Geometry: final body of the model. Coordinates: model frame, mm. A direction names the side the tool comes from. Give positions to 0.01 mm unless a question says otherwise; leave off trailing zeros. Loops run counter-clockwise (first coordinate to the right, second up) from the corner with the lowest first, then second, coordinate; pieces in that order, holes last. Notation, with made-up numbers: (-14, -25) -> (40, -25) arc R28 ccw to (40, 8) -> close; hole circle Ø6 at (-38, 28.5). An arc over 180 degrees is marked (long way). Answer in a Markdown table with one row per item. Add a question column.
1) Line query: line 1 (X direction, y = 10, z = 15.5); line 2 (X direction, y = 3.5, z = 10.25); line 3 (Y direction, x = -108.75, z = 9.75). Output: solid intervals per line, ascending. Write a range as from..to.
2) First-contact query: P1, Ø3, axis at x = -49, y = 33.5, coming from the -Z side; P2, Ø4.5, axis at x = -108.75, y = 10, coming from the +Z side; P3, Ø8, axis at x = -129.5, z = 9.5, coming from the +Y side. Flat tips, straight axial feed; report the tip coordinate or a pass-through.
3) Section query A-A (z = 1.75). Return the cut outline in (x, y), plus the area to 3 significant figures.
4) Section query B-B (x = -108.75). Return the cut outline in (y, z), plus the area to 3 significant figures.
5) Access query for faces 1 (the flat face through (-74, 0, 10)), 2 (the cylindrical face through (-92.73, 0.52, 10.14)). Directions: +Z, -Z, +X, -X, +Y, -Y. A direction counts if a zero-diameter tool reaches every point of the face in a straight line with its end or side. Return the directions, or none.
6) Section query C-C (y = 25). Return the cut outline in (x, z).
7) Section query D-D (x = -40). Return the cut outline in (y, z).
Autodesk Inventor part; units mm, degrees
ref_plane "YZ Plane" through (0, 0, 0) normal (1, 0, 0) x (0, 1, 0)
ref_plane "XZ Plane" through (0, 0, 0) normal (0, 1, 0) x (-1, 0, 0)
ref_plane "XY Plane" through (0, 0, 0) normal (0, 0, 1) x (1, 0, 0)
sketch "Sketch1" plane through (0, 0, 0) normal (0, 0, 1) x (1, 0, 0)
  line L0 (0, 0) -> (-48.9676, 0)
  line L1 (-147.5, 0) -> (-147.5, 20.4375)
  line L2 (-147.5, 40) -> (-73.75, 40)
  line L3 (0, 40) -> (0, 30.4375)
  line L4 (-108.75, 10) -> (-38.75, 10)
  line L5 (-108.75, 10) -> (-117.5, 10)
  line L6 (-38.75, 10) -> (-30, 10)
  line L7 (-98.9676, 0) -> (-92.4032, 0)
  line L8 (-147.5, 0) -> (-98.9676, 0)
  line L9 (-48.9676, 0) -> (0, 0)
  line L10 (-147.5, 10) -> (-117.5, 10)
  line L11 (0, 10) -> (-30, 10)
  line L12 (-98.9676, 0) -> (-117.5, 10)
  line L13 (-48.9676, 0) -> (-30, 10)
  line L14 (-117.5, 10) -> (-147.5, 10)
  line L15 (-30, 10) -> (0, 10)
  circle A0 centre (-108.75, 10) radius 2.5
  circle A1 centre (-38.75, 10) radius 2.5
  line L16 (-147.5, 10) -> (-147.5, 20.4375)
  line L17 (-117.5, 10) -> (-147.5, 20.4375)
  line L18 (0, 10) -> (0, 20.4375)
  line L19 (0, 20.4375) -> (-147.5, 20.4375)
  line L20 (-30, 10) -> (0, 20.4375)
  line L21 (-147.5, 20.4375) -> (-147.5, 30.4375)
  line L22 (-147.5, 30.4375) -> (-73.75, 40)
  line L23 (0, 20.4375) -> (0, 30.4375)
  line L24 (-73.75, 40) -> (0, 30.4375)
  line L25 (0, 20.4375) -> (0, 0)
  line L26 (0, 30.4375) -> (0, 20.4375)
  line L27 (-147.5, 30.4375) -> (-147.5, 40)
  line L28 (-147.5, 20.4375) -> (-147.5, 30.4375)
  line L29 (-73.75, 40) -> (0, 40)
  line L30 (-88.7871, 0) -> (-58.7871, 0)
  line L31 (-88.7575, 0) -> (-58.7871, 0)
  line L32 (-88.7575, 0) -> (-88.7575, 6.2461)
  line L33 (-58.7871, 0) -> (-58.7871, 7.0063)
  line L34 (-58.7871, 7.0063) -> (-62.8766, 0)
  line L35 (-58.7871, 7.0063) -> (-55.532, 0)
  line L36 (-88.7575, 6.2461) -> (-85.8556, 0)
  line L37 (-88.7575, 6.2461) -> (-92.4032, 0)
  line L38 (-58.7871, 0) -> (-55.532, 0)
  line L39 (-92.4032, 0) -> (-147.5, 0)
  line L40 (-48.9676, 0) -> (-55.532, 0)
  line L41 (-55.532, 0) -> (-92.4032, 0)
  line L42 (-92.4032, 0) -> (-88.7575, 0)
  line L43 (-55.532, 0) -> (-48.9676, 0)
  point P0 (-73.75, 0)
  point P1 (-85.8556, 0)
  dimension "d0" = 147.5
  dimension "d1" = 40
  dimension "d2" = 70
  dimension "d3" = 10
  dimension "d4" = 50
  dimension "d5" = 30
  dimension "d6" = 30
  dimension "d7" = 5
  dimension "d8" = 5
  dimension "d9" = 10
  dimension "d10" = 30
extrude "Extrusion2" add sketch "Sketch1" along normal blind 20 contours L40 L35 L34 L30 L36 L37 L7 L12 L5 A0 L4 A1 L6 L13 | L6 A1 L4 A0 L5 L17 L19 L20 | L19 L21 L22 L24 L23
fillet "Fillet5" radius 100 1 edges at (-73.75, 40, 10)
fillet "Fillet6" radius 15 2 edges at (0, 30.4375, 10) (-147.5, 30.4375, 10)
fillet "Fillet7" radius 10 2 edges at (-117.5, 10, 10) (-30, 10, 10)
fillet "Fillet8" radius 4 6 edges at (-98.9676, 0, 10) (-92.4032, 0, 10) (-55.532, 0, 10) (-48.9676, 0, 10) (-85.8556, 0, 10) (-62.8766, 0, 10)
fillet "Fillet9" radius 2 2 edges at (-88.7575, 6.2461, 10) (-58.7871, 7.0063, 10)
properties part number "bumper" material "Polystyrene, Expanded"
Evaluation:
| question | item | result |
|---|---|---|
| 1 | line 1 | -117.58..-111.25, -106.25..-41.25, -36.25..-29.93 |
| 1 | line 2 | -105.45..-90.2, -87.72..-60.83, -57.16..-42.33 |
| 1 | line 3 | 5.28..7.5, 12.5..35.46 |
| 2 | P1 | z = 0 |
| 2 | P2 | through |
| 2 | P3 | y = 33.29 |
| 3 | outline | (-147.5, 20.44) -> (-118.26, 10.26) arc R10 cw to (-116.79, 9.62) -> (-99.86, 0.48) arc R4 ccw to (-97.96, 0) -> (-94.7, 0) arc R4 ccw to (-91.25, 1.98) -> (-90.69, 2.94) arc R2 cw to (-87.15, 2.78) -> (-86.93, 2.31) arc R4 ccw to (-83.3, 0) -> (-65.17, 0) arc R4 ccw to (-61.72, 1.98) -> (-60.72, 3.7) arc R2 cw to (-57.17, 3.54) -> (-56.61, 2.31) arc R4 ccw to (-52.98, 0) -> (-49.96, 0) arc R4 ccw to (-48.09, 0.46) -> (-30.67, 9.65) arc R10 cw to (-29.29, 10.25) -> (0, 20.44) arc R15 ccw to (-12.72, 32.09) -> (-60.89, 38.33) arc R100 ccw to (-86.61, 38.33) -> (-134.78, 32.09) arc R15 ccw to start; hole circle Ø5 at (-108.75, 10); hole circle Ø5 at (-38.75, 10) |
| 3 | area | 3,940 mm² |
| 4 | outline | (5.28, 0) -> (7.5, 0) -> (7.5, 20) -> (5.28, 20) -> close; (12.5, 0) -> (35.46, 0) -> (35.46, 20) -> (12.5, 20) -> close |
| 4 | area | 504 mm² |
| 5 | face 1 | +Z, -Z, +X, -X, -Y |
| 5 | face 2 | +Z, -Z, -Y |
| 6 | outline | (-145.67, 0) -> (-1.83, 0) -> (-1.83, 20) -> (-145.67, 20) -> close |
| 7 | outline | (4.73, 0) -> (7.83, 0) -> (7.83, 20) -> (4.73, 20) -> close; (12.17, 0) -> (35.62, 0) -> (35.62, 20) -> (12.17, 20) -> close |
